The model under review builds one solid part; all positions refer to its coordinate system, in mm. Face numbers are marked on the shaded views. A direction names the side the tool comes from. Coordinates: 2 decimals unless noted, no trailing zeros. Loops run counter-clockwise (first coordinate to the right, second up) from the corner with the lowest first, then second, coordinate; pieces in that order, holes last. Notation, with made-up numbers: M 66.25,-37.5 L 114.25,-37.5 A14 cw 114.25,-20.5 Z; hole C 4.25,43 d7. An arc over 180 degrees is marked long. Return JSON: item names as keys, results as strings.
```python
from build123d import *

# Parameters (mm, degrees)
SKETCH6_W       = 12.319
SKETCH6_H       = 1.778
SLOT_DEPTH      = 1.4478
THDSCHPAT_COUNT = 16
THDSCHPAT_PITCH = 1.27


with BuildPart() as part:
    # BodySke → Base-Revolve (revolve)
    with BuildSketch(Plane.XY):
        Polygon((0, 0), (0, 6.1595), (0.122725489, 6.1595), (3.556, 3.175), (25.4, 3.175), (25.4, 0), align=None)
    revolve(axis=Axis((-6.35, 0, 0), (1, 0, 0)))

    # Sketch6 → Slot (cut)
    with BuildSketch(Plane.ZY):
        Rectangle(SKETCH6_W, SKETCH6_H)
    extrude(amount=-SLOT_DEPTH, mode=Mode.SUBTRACT)

    # ThdSchSke → ThreadSchematic (revolve, cut)
    with BuildSketch(Plane.XY):
        Polygon((6.3500254, -2.41935), (5.820913574, -3.175), (5.820913574, -3.96875), (6.879137226, -3.96875), (6.879137226, -3.175), align=None)
    threadschematic = revolve(axis=Axis((-3.175, 0, 0), (1, 0, 0)), mode=Mode.SUBTRACT)

    # ThdSchPat: ThreadSchematic ×16
    with Locations(*[(i * THDSCHPAT_PITCH, 0, 0) for i in range(1, THDSCHPAT_COUNT)]):
        add(threadschematic, mode=Mode.SUBTRACT)


solid = part.part
```
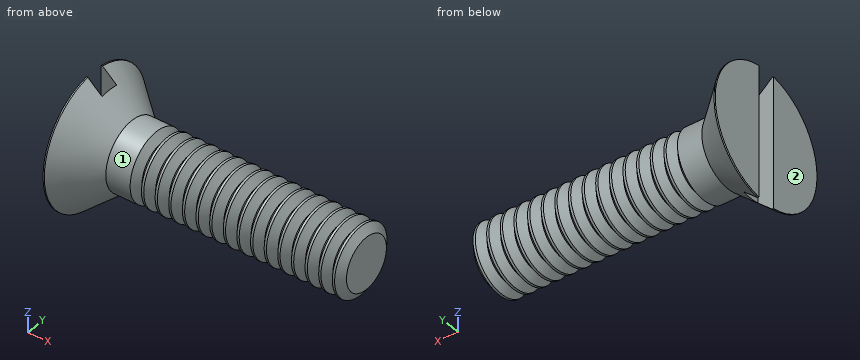
1. To check wall thickness, follow line 1 (X direction, y = -3.25, z = 0.75); line 2 (X direction, y = -2.25, z = -5.5); line 3 (Y direction, x = 4.75, z = -1.5). State the ranges of each line that lie inside material, in increasing order.
Check values:
{"line 1": "0 to 3.37", "line 2": "0 to 0.37", "line 3": "-2.8 to 2.8"}
2. Insertion check: pin 1 Ø5 at (x, z) = (19.5, -3) entering from -Y; pin 2 Ø3 at (x, y) = (21.5, 2.5) entering from -Z; pin 3 Ø1.4 at (y, z) = (0, 1.5) entering from -X. Each pin has a flat end and moves straight along its axis. Give the tip position at first contact, or say it passes through.
Check values:
{"pin 1": "y = -3.14", "pin 2": "z = -2.99", "pin 3": "x = 1.45"}
3. Add section A-A on x = 4.75. Give the boundary of the cut face in (y, z) (3 decimals), plus the area to 3 significant figures.
Check values:
{"outline": "C 0,0 d6.35", "area": "31.7 mm²"}
4. Add section B-B on y = -2.75. State how many separate pieces and enclosed holes the cut face has, plus the area to 3 significant figures.
Check values:
{"separate pieces": "16", "enclosed holes": "0", "area": "63.3 mm²"}
5. Machinability: for the marked faces 1 and 2, which of the approach directions +Z, -Z, +X, -X, +Y, -Y give a long, thin tool a straight path to every point of the face, cutting with its end or side? Answer none if there is none.
Check values:
{"face 1": "+X", "face 2": "+Z, -Z, -X, +Y, -Y"}
